The listing builds one solid part. Answer for the finished solid, in the listing's coordinates (mm). Face numbers are marked on the shaded views. Round coordinates to 2 decimals unless told otherwise and drop trailing zeros. Loops run counter-clockwise (first coordinate to the right, second up) from the corner with the lowest first, then second, coordinate; pieces in that order, holes last. Notation, with made-up numbers: (45.5, 72) -> (60.5, 72) arc R5 ccw to (60.5, 81) -> close; hole circle Ø4 at (-33, -14). An arc over 180 degrees is marked (long way). Answer in a Markdown table with one row per item. Add a question column.
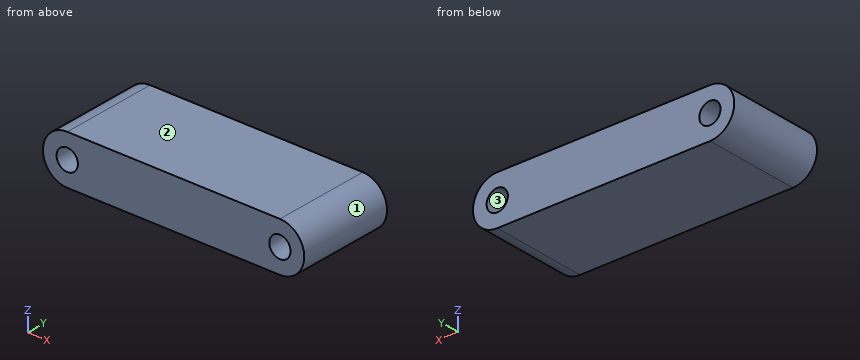
Autodesk Inventor part; units mm, degrees
ref_plane "YZ Plane" through (0, 0, 0) normal (1, 0, 0) x (0, 1, 0)
ref_plane "XZ Plane" through (0, 0, 0) normal (0, 1, 0) x (-1, 0, 0)
ref_plane "XY Plane" through (0, 0, 0) normal (0, 0, 1) x (1, 0, 0)
sketch "Sketch1" plane through (0, 0, 0) normal (0, 1, 0) x (-1, 0, 0)
  line L0 (-27.7812, 0) -> (27.7812, 0) construction
  line L1 (-27.7812, -6.35) -> (27.7812, -6.35)
  line L2 (27.7812, 6.35) -> (-27.7812, 6.35)
  arc A0 (-27.7812, 6.35) -> (-27.7812, -6.35) centre (-27.7812, 0) ccw
  arc A1 (27.7812, -6.35) -> (27.7812, 6.35) centre (27.7812, 0) ccw
  circle A2 centre (27.7812, 0) radius 2.7781
  circle A3 centre (-27.7812, 0) radius 2.7781
  point P0 (0, 0)
  dimension "d0" = 5.5563
  dimension "d1" = 55.5625
  dimension "d2" = 6.35
extrude "Extrusion1" add sketch "Sketch1" along normal blind 25.4
properties part number "OZZ-CasterRiserBlock" material "Steel, Alloy"
Item 1: Section B-B, the plane y = 3 is taken. Write down the section's boundary in (x, z), and give its area (3 significant figures).
Item 2: Consider L1, parallel to X at y = 9.5, z = -2.25; L2, parallel to X at y = 19.25, z = -2; L3, parallel to Z at x = 27, y = 23.5. Determine where each line is inside the solid, lowest interval first. Write a range as from..to.
Item 3: Section D-D, the plane z = -4.25 is taken. Write down the section's boundary in (x, y), and give its area (3 significant figures).
Item 4: The mould has two halves that part along X. Classify the marked faces 1, 2 and 3: +X half, -X half, draft (parallel to the pull), parting line (faces both ways), or undercut.
Item 5: Section C-C, the plane x = 27 is taken. Write down the section's boundary in (y, z), and give its area (3 significant figures).
Item 6: Section A-A, the plane z = 0 is taken. Write down the section's boundary in (x, y).
Item 7: Flat-ended cylindrical pins translate along their axes: P1, Ø6, axis at y = 22.5, z = -0.5, coming from the -X side; P2, Ø1.5, axis at y = 14.5, z = 4, coming from the -X side; P3, Ø1, axis at y = 12, z = -1.5, coming from the +X side. Find the tip coordinate at first contact, or state that the pin passes through.
Here are the results:
| question | item | result |
|---|---|---|
| 1 | outline | (-27.78, -6.35) -> (27.78, -6.35) arc R6.35 ccw to (27.78, 6.35) -> (-27.78, 6.35) arc R6.35 ccw to start; hole circle Ø5.56 at (-27.78, 0); hole circle Ø5.56 at (27.78, 0) |
| 1 | area | 784 mm² |
| 2 | L1 | x = -33.72..-29.41, -26.15..26.15, 29.41..33.72 |
| 2 | L2 | x = -33.81..-29.71, -25.85..25.85, 29.71..33.81 |
| 2 | L3 | z = -6.35..-2.67, 2.67..6.35 |
| 3 | outline | (-32.5, 0) -> (32.5, 0) -> (32.5, 25.4) -> (-32.5, 25.4) -> close |
| 3 | area | 1,650 mm² |
| 4 | face 1 | +X half |
| 4 | face 2 | draft |
| 4 | face 3 | undercut |
| 5 | outline | (0, -6.35) -> (25.4, -6.35) -> (25.4, -2.67) -> (0, -2.67) -> close; (0, 2.67) -> (25.4, 2.67) -> (25.4, 6.35) -> (0, 6.35) -> close |
| 5 | area | 187 mm² |
| 6 | outline | (-34.13, 0) -> (-30.56, 0) -> (-30.56, 25.4) -> (-34.13, 25.4) -> close; (-25, 0) -> (25, 0) -> (25, 25.4) -> (-25, 25.4) -> close; (30.56, 0) -> (34.13, 0) -> (34.13, 25.4) -> (30.56, 25.4) -> close |
| 7 | P1 | stops at x = -34.13 |
| 7 | P2 | stops at x = -33.24 |
| 7 | P3 | stops at x = 34.05 |
